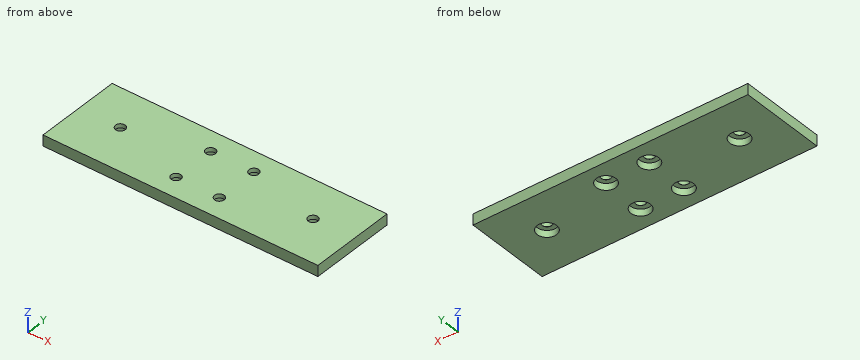
from build123d import *

# Parameters (mm, degrees)
ESQUISSE1_W                                  = 127
ESQUISSE1_H                                  = 40
BOSS_EXTRU_1_DEPTH                           = 5
CHAMBRAGE_POUR_VIS_T_TE_RONDE_BOMB_2_COUNT   = 2
CHAMBRAGE_POUR_VIS_T_TE_RONDE_BOMB_2_PITCH   = 89
D_GAGEMENT_M21_D                             = 2.4
CHAMBRAGE_POUR_VIS_T_TE_RONDE_BOMB_3_A_COUNT = 2
CHAMBRAGE_POUR_VIS_T_TE_RONDE_BOMB_3_A_PITCH = 20
CHAMBRAGE_POUR_VIS_T_TE_RONDE_BOMB_4_COUNT   = 2
CHAMBRAGE_POUR_VIS_T_TE_RONDE_BOMB_4_PITCH   = 20
CHAMBRAGE_POUR_VIS_T_TE_RONDE_BOMB_5_COUNT   = 2
CHAMBRAGE_POUR_VIS_T_TE_RONDE_BOMB_5_PITCH   = 28.284271247


with BuildPart() as part:
    # Esquisse1 → Boss.-Extru.1 (new body)
    with BuildSketch(Plane.XY):
        Rectangle(ESQUISSE1_W, ESQUISSE1_H)
    extrude(amount=BOSS_EXTRU_1_DEPTH)

    # Esquisse2 → Chambrage pour vis _ t_te ronde bomb_e M (revolve, cut)
    with BuildSketch(Plane(origin=(44.5, 1, 0), x_dir=(0, 1, 0), z_dir=(1, 0, 0))):
        Polygon((0, 0), (0, 5), (2.25, 5), (2.25, 3.125), (2.275, 3.1), (4.5, 3.1), (4.5, 0), align=None)
    chambrage_pour_vis_t_te_ronde_bomb_e_m = revolve(axis=Axis((44.5, 1, -6.35), (0, 0, 1)), mode=Mode.SUBTRACT)

    # Chambrage pour vis _ t_te ronde bomb 2: Chambrage pour vis _ t_te ronde bomb_e M ×2
    with Locations(*[(-i * CHAMBRAGE_POUR_VIS_T_TE_RONDE_BOMB_2_PITCH, 0, 0) for i in range(1, CHAMBRAGE_POUR_VIS_T_TE_RONDE_BOMB_2_COUNT)]):
        add(chambrage_pour_vis_t_te_ronde_bomb_e_m, mode=Mode.SUBTRACT)

    # Dégagement M21 (through all)
    with Locations(Plane.XY.offset(5)):
        with Locations((10, -10), (10, 10), (-10, -10), (-10, 10)):
            Hole(D_GAGEMENT_M21_D / 2)

    # Esquisse6 → Chambrage pour vis _ t_te ronde bomb 3 (revolve, cut)
    with BuildSketch(Plane(origin=(10, -10, 0), x_dir=(0, 1, 0), z_dir=(1, 0, 0))):
        Polygon((0, 0), (0, 5), (2.25, 5), (2.25, 3.125), (2.275, 3.1), (4.5, 3.1), (4.5, 0), align=None)
    chambrage_pour_vis_t_te_ronde_bomb_3 = revolve(axis=Axis((10, -10, -6.35), (0, 0, 1)), mode=Mode.SUBTRACT)

    # Chambrage pour vis _ t_te ronde bomb 3 a: Chambrage pour vis _ t_te ronde bomb 3 ×2
    with Locations(*[(0, i * CHAMBRAGE_POUR_VIS_T_TE_RONDE_BOMB_3_A_PITCH, 0) for i in range(1, CHAMBRAGE_POUR_VIS_T_TE_RONDE_BOMB_3_A_COUNT)]):
        add(chambrage_pour_vis_t_te_ronde_bomb_3, mode=Mode.SUBTRACT)

    # Chambrage pour vis _ t_te ronde bomb 4: Chambrage pour vis _ t_te ronde bomb 3 ×2
    with Locations(*[(-i * CHAMBRAGE_POUR_VIS_T_TE_RONDE_BOMB_4_PITCH, 0, 0) for i in range(1, CHAMBRAGE_POUR_VIS_T_TE_RONDE_BOMB_4_COUNT)]):
        add(chambrage_pour_vis_t_te_ronde_bomb_3, mode=Mode.SUBTRACT)

    # Chambrage pour vis _ t_te ronde bomb 5: Chambrage pour vis _ t_te ronde bomb 3 ×2
    with Locations(*[Vector(-0.7071067811865411, 0.707106781186554, 0) * (i * CHAMBRAGE_POUR_VIS_T_TE_RONDE_BOMB_5_PITCH) for i in range(1, CHAMBRAGE_POUR_VIS_T_TE_RONDE_BOMB_5_COUNT)]):
        add(chambrage_pour_vis_t_te_ronde_bomb_3, mode=Mode.SUBTRACT)


solid = part.part
Verification items for the finished model (mm, model axes). Coordinates: 2 decimals unless noted, no trailing zeros. Loops run counter-clockwise (first coordinate to the right, second up) from the corner with the lowest first, then second, coordinate; pieces in that order, holes last. Notation, with made-up numbers: (63.5, 17.25) -> (118.5, 17.25) arc R19 ccw to (118.5, 44.25) -> close; hole circle Ø1 at (5.5, 67.5). An arc over 180 degrees is marked (long way). Answer as a JSON object with one key per item and string values. Group by question number.
Item 1: Sectioned sample at D-D on x = 44.5. Record the boundary of the cut face in (y, z) (3 decimals), plus the area to 3 significant figures.
Item 2: Sectioned sample at A-A on x = 10. Record the boundary of the cut face in (y, z) (3 decimals), plus the area to 3 significant figures.
Item 3: Sectioned sample at B-B on y = -10. Record the boundary of the cut face in (x, z) (3 decimals), plus the area to 3 significant figures.
Item 4: Sectioned sample at C-C on z = 1.9. Record the boundary of the cut face in (x, y), plus the area to 3 significant figures.
Item 5: Scan lines: probe 1 along X at (y, z) = (1, 2.3); probe 2 along Y at (x, z) = (10, 2.3); probe 3 along X at (y, z) = (1, 4.35). Record each from-to range of solid material in increasing order.
Item 6: Depth check by flat-ended pin: pin 1 (8 mm diameter, centred on x = -10, y = 10, fed in from -Z); pin 2 (3.5 mm diameter, centred on x = -10, y = -10, fed in from -Z). Enter the tip coordinate at first touch or a pass-through.
Evaluation:
{
 "1": {"outline": "(-20, 0) -> (-3.5, 0) -> (-3.5, 3.1) -> (-1.275, 3.1) -> (-1.25, 3.125) -> (-1.25, 5) -> (-20, 5) -> close; (3.25, 3.125) -> (3.275, 3.1) -> (5.5, 3.1) -> (5.5, 0) -> (20, 0) -> (20, 5) -> (3.25, 5) -> close", "area": "164 mm²"},
 "2": {"outline": "(-20, 0) -> (-14.5, 0) -> (-14.5, 3.1) -> (-12.275, 3.1) -> (-12.25, 3.125) -> (-12.25, 5) -> (-20, 5) -> close; (-7.75, 3.125) -> (-7.725, 3.1) -> (-5.5, 3.1) -> (-5.5, 0) -> (5.5, 0) -> (5.5, 3.1) -> (7.725, 3.1) -> (7.75, 3.125) -> (7.75, 5) -> (-7.75, 5) -> close; (12.25, 3.125) -> (12.275, 3.1) -> (14.5, 3.1) -> (14.5, 0) -> (20, 0) -> (20, 5) -> (12.25, 5) -> close", "area": "127 mm²"},
 "3": {"outline": "(-63.5, 0) -> (-14.5, 0) -> (-14.5, 3.1) -> (-12.275, 3.1) -> (-12.25, 3.125) -> (-12.25, 5) -> (-63.5, 5) -> close; (-7.75, 3.125) -> (-7.725, 3.1) -> (-5.5, 3.1) -> (-5.5, 0) -> (5.5, 0) -> (5.5, 3.1) -> (7.725, 3.1) -> (7.75, 3.125) -> (7.75, 5) -> (-7.75, 5) -> close; (12.25, 3.125) -> (12.275, 3.1) -> (14.5, 3.1) -> (14.5, 0) -> (63.5, 0) -> (63.5, 5) -> (12.25, 5) -> close", "area": "562 mm²"},
 "4": {"outline": "(-63.5, -20) -> (63.5, -20) -> (63.5, 20) -> (-63.5, 20) -> close; hole circle Ø9 at (-44.5, 1); hole circle Ø9 at (-10, -10); hole circle Ø9 at (-10, 10); hole circle Ø9 at (10, -10); hole circle Ø9 at (10, 10); hole circle Ø9 at (44.5, 1)", "area": "4,700 mm²"},
 "5": {"probe 1": "x = -63.5 to -49, -40 to 40, 49 to 63.5", "probe 2": "y = -20 to -14.5, -5.5 to 5.5, 14.5 to 20", "probe 3": "x = -63.5 to -46.75, -42.25 to 42.25, 46.75 to 63.5"},
 "6": {"pin 1": "stops at z = 3.1", "pin 2": "passes through"}
}
